CAD build for the part. Positions are in the model's coordinates, mm. Coordinates: 2 decimals unless noted, no trailing zeros. Loops run counter-clockwise (first coordinate to the right, second up) from the corner with the lowest first, then second, coordinate; pieces in that order, holes last. Notation, with made-up numbers: (-36, 1) -> (-24, 1) arc R29 ccw to (-24, 26) -> close; hole circle Ø7 at (51, -24.5). An arc over 180 degrees is marked (long way). Write each question's results on one line, items separated by ' | '.
```python
from build123d import *

# Parameters (mm, degrees)
SKETCH1_R           = 1.65
BOSS_EXTRUDE1_DEPTH = 6
FILLET1_R           = 5
SKETCH2_R           = 5.1
CUT_EXTRUDE1_DEPTH  = 157.355060824


with BuildPart() as part:
    # Sketch1 → Boss-Extrude1 (new body)
    with BuildSketch(Plane(origin=(0, 0, 0), x_dir=(1, 0, 0), z_dir=(0, 1, 0))):
        with BuildLine():
            ThreePointArc((-111.234035703, -19.613561667), (-112.95, 0), (-111.234035703, 19.613561667))
            ThreePointArc((-111.234035703, 19.613561667), (-109.13025705, 22.87401705), (-105.327953741, 23.647931427))
            ThreePointArc((-105.327953741, 23.647931427), (0, 107.95), (105.327953741, 23.647931427))
            ThreePointArc((105.327953741, 23.647931427), (109.13025705, 22.87401705), (111.234035703, 19.613561667))
            ThreePointArc((111.234035703, 19.613561667), (112.95, 0), (111.234035703, -19.613561667))
            ThreePointArc((111.234035703, -19.613561667), (109.13025705, -22.87401705), (105.327953741, -23.647931427))
            ThreePointArc((105.327953741, -23.647931427), (0, -107.95), (-105.327953741, -23.647931427))
            ThreePointArc((-105.327953741, -23.647931427), (-109.13025705, -22.87401705), (-111.234035703, -19.613561667))
        make_face()
        with Locations(Location((0, 104.55, 0), (0, 0, 270))):
            Circle(SKETCH1_R, mode=Mode.SUBTRACT)
        with Locations(Location((52.275, 90.542955966, 0), (0, 0, 270))):
            Circle(SKETCH1_R, mode=Mode.SUBTRACT)
        with Locations(Location((90.542955966, 52.275, 0), (0, 0, 270))):
            Circle(SKETCH1_R, mode=Mode.SUBTRACT)
        with Locations(Location((104.55, 0, 0), (0, 0, 270))):
            Circle(SKETCH1_R, mode=Mode.SUBTRACT)
        with Locations(Location((90.542955966, -52.275, 0), (0, 0, 270))):
            Circle(SKETCH1_R, mode=Mode.SUBTRACT)
        with Locations(Location((52.275, -90.542955966, 0), (0, 0, 270))):
            Circle(SKETCH1_R, mode=Mode.SUBTRACT)
        with Locations(Location((0, -104.55, 0), (0, 0, 270))):
            Circle(SKETCH1_R, mode=Mode.SUBTRACT)
        with Locations(Location((-52.275, -90.542955966, 0), (0, 0, 270))):
            Circle(SKETCH1_R, mode=Mode.SUBTRACT)
        with Locations(Location((-90.542955966, -52.275, 0), (0, 0, 270))):
            Circle(SKETCH1_R, mode=Mode.SUBTRACT)
        with Locations(Location((-104.55, 0, 0), (0, 0, 270))):
            Circle(SKETCH1_R, mode=Mode.SUBTRACT)
        with Locations(Location((-90.542955966, 52.275, 0), (0, 0, 270))):
            Circle(SKETCH1_R, mode=Mode.SUBTRACT)
        with Locations(Location((-52.275, 90.542955966, 0), (0, 0, 270))):
            Circle(SKETCH1_R, mode=Mode.SUBTRACT)
    extrude(amount=BOSS_EXTRUDE1_DEPTH)

    # Fillet1
    fillet1_edges = [part.edges().sort_by_distance(p)[0] for p in [
        (-105.327953741, 3, -23.647931427),
        (105.327953741, 3, -23.647931427),
        (105.327953741, 3, 23.647931427),
        (-105.327953741, 3, 23.647931427),
    ]]
    fillet(fillet1_edges, radius=FILLET1_R)

    # Sketch2 → Cut-Extrude1 (cut, through all)
    with BuildSketch(Plane(origin=(0, 6, 0), x_dir=(1, 0, 0), z_dir=(0, 1, 0))):
        with Locations(Location((0, 53.975, 0), (0, 0, 270))):
            Circle(SKETCH2_R)
        with Locations(Location((51.333275467, 16.679192271, 0), (0, 0, 270))):
            Circle(SKETCH2_R)
        with Locations(Location((31.725708992, -43.666692271, 0), (0, 0, 270))):
            Circle(SKETCH2_R)
        with Locations(Location((-31.725708992, -43.666692271, 0), (0, 0, 270))):
            Circle(SKETCH2_R)
        with Locations(Location((-51.333275467, 16.679192271, 0), (0, 0, 270))):
            Circle(SKETCH2_R)
    extrude(amount=-CUT_EXTRUDE1_DEPTH, mode=Mode.SUBTRACT)


solid = part.part
```
Q1. Cut at C-C on x = -19.5. Write the cut outline in (y, z), and give its area (3 significant figures).
Results are:
outline: (0, -106.17) -> (6, -106.17) -> (6, 106.17) -> (0, 106.17) -> close | area: 1,270 mm^2
Q2. Wall check: L1, parallel to X at y = 1, z = 47; L2, parallel to X at y = 1.25, z = -12.5; L3, parallel to Z at x = 19, y = 5.75. Give the ranges that are in metal, low to high. Write a range as from..to.
Results are:
L1: -97.18..-35.59, -27.87..27.87, 35.59..97.18 | L2: -112.26..-54.26, -48.41..48.41, 54.26..112.26 | L3: -106.26..106.26
Q3. Pull direction Z, two halves, no side cores. Call faces 1 (the cylindrical face through (112.95, 2.96, -0.28)), 2 (the flat face through (2, 6, -2)), 3 (the cylindrical face through (-30.19, 3.04, 48.53)): +Z half, -Z half, draft (parallel to the pull), parting line (faces both ways), or undercut.
Results are:
face 1: parting line | face 2: draft | face 3: undercut
Q4. Cut at B-B on z = 78.5. Write the cut outline in (x, y).
Results are:
outline: (-74.1, 0) -> (74.1, 0) -> (74.1, 6) -> (-74.1, 6) -> close
Q5. Cut at A-A on y = 4.5. Give the number of separate pieces and of enclosed holes in the cut face, and give its area (3 significant figures).
Results are:
separate pieces: 1 | enclosed holes: 17 | area: 36,600 mm^2
Q6. Drop flat-ended pins along their axis: pin 1 (1.5 mm diameter, centred on y = 5, z = 39, fed in from +X); pin 2 (1.5 mm diameter, centred on x = 56.5, z = -23.5, fed in from -Y); pin 3 (6 mm diameter, centred on x = -31.73, z = 43.67, fed in from +Y); pin 4 (2 mm diameter, centred on x = -52.5, y = 5, fed in from -Z). Give the stop position or say it passes through.
Results are:
pin 1: x = 100.95 | pin 2: y = 0 | pin 3: through | pin 4: z = -94.87
